Work out the finished part from the listing and answer in its coordinate system (mm). Give positions to 0.01 mm unless a question says otherwise; leave off trailing zeros. Loops run counter-clockwise (first coordinate to the right, second up) from the corner with the lowest first, then second, coordinate; pieces in that order, holes last. Notation, with made-up numbers: (60.5, 31.5) -> (101.5, 31.5) arc R26 cw to (101.5, 57.5) -> close; hole circle Ø7 at (-13, -32.5). An arc over 180 degrees is marked (long way). Answer as CSV lines item,"result". Start each with the question number.
1. Find section B-B, the plane y = 14.75. Give the vertices of the cut face in (x, z).
2. Find section A-A, the plane z = 232.5. Give the vertices of the cut face in (x, y).
3. Flat-ended cylindrical pins translate along their axes: pin 1 Ø1.7 at (y, z) = (10, 272) entering from -X; pin 2 Ø7 at (y, z) = (8, 477) entering from -X; pin 3 Ø1.5 at (y, z) = (2.5, 426) entering from -X; pin 4 Ø4 at (x, z) = (-6, 469) entering from +Y. Find the tip coordinate at first contact, or state that the pin passes through.
4. Find the intervals of material crossed by line 1 along Z through (x, y) = (-1.75, 10.5); line 2 along Y through (x, z) = (-1.3, 136); line 3 along Z through (x, y) = (-2.25, 9.25), in increasing order.
from build123d import *

# Parameters (mm, degrees)
EXTRUDE_1_DEPTH      = 680
HOLE_WIZARD_M3_5_1_D = 2.9
FILLET_1_R           = 1
FILLET_2_R           = 0.5


with BuildPart() as part:
    # 草图1 → 凸台-拉伸1 (new body)
    with BuildSketch(Plane.XY):
        Polygon((0, 0), (0, 18), (-2.5, 18), (-2.5, 2), (-7.5, 2), (-7.5, 0), align=None)
    extrude(amount=EXTRUDE_1_DEPTH)

    # M3.5 螺纹孔1 (through all)
    with Locations(Plane.ZY.offset(2.5)):
        with Locations((136, 10), (272, 10), (408, 10), (544, 10)):
            Hole(HOLE_WIZARD_M3_5_1_D / 2)

    # 圆角1
    fillet_1_edges = [part.edges().sort_by_distance(p)[0] for p in [
        (-2.5, 2, 340),
        (0, 0, 340),
    ]]
    fillet(fillet_1_edges, radius=FILLET_1_R)

    # 圆角2
    fillet_2_edges = [part.edges().sort_by_distance(p)[0] for p in [
        (-7.5, 0, 340),
        (-7.5, 2, 340),
        (-2.5, 18, 340),
        (0, 18, 340),
        (-7.5, 1, 680),
        (-7.5, 1, 0),
    ]]
    fillet(fillet_2_edges, radius=FILLET_2_R)


solid = part.part
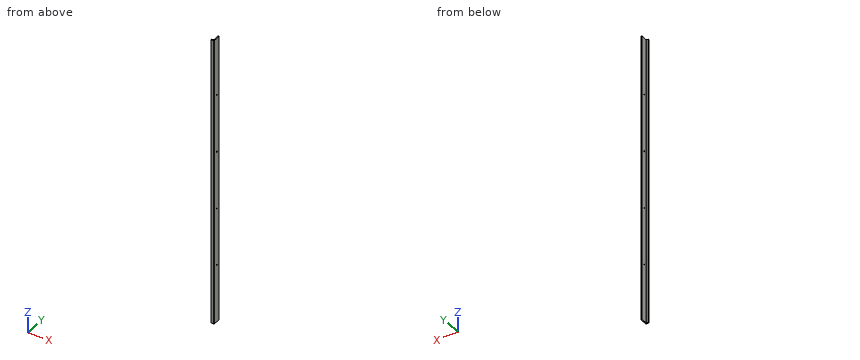
Resolved:
1,outline,"(-2.5, 0) -> (0, 0) -> (0, 680) -> (-2.5, 680) -> close"
2,outline,"(-7.5, 0.5) arc R0.5 ccw to (-7, 0) -> (-1, 0) arc R1 ccw to (0, 1) -> (0, 17.5) arc R0.5 ccw to (-0.5, 18) -> (-2, 18) arc R0.5 ccw to (-2.5, 17.5) -> (-2.5, 3) arc R1 cw to (-3.5, 2) -> (-7, 2) arc R0.5 ccw to (-7.5, 1.5) -> close"
3,pin 1,"passes through"
3,pin 2,"stops at x = -2.5"
3,pin 3,"stops at x = -7.43"
3,pin 4,"stops at y = 2"
4,line 1,"z = 0 to 134.64, 137.36 to 270.64, 273.36 to 406.64, 409.36 to 542.64, 545.36 to 680"
4,line 2,"y = 0 to 8.55, 11.45 to 18"
4,line 3,"z = 0 to 134.76, 137.24 to 270.76, 273.24 to 406.76, 409.24 to 542.76, 545.24 to 680"
